from build123d import *

# Parameters (mm, degrees)
SKETCH1_W                                     = 127
SKETCH1_H                                     = 190.5
BOSS_EXTRUDE1_DEPTH                           = 16
SKETCH3_W                                     = 73.2
SKETCH3_H                                     = 190.5
CUT_EXTRUDE2_DEPTH                            = 14
SKETCH6_W                                     = 73.2
SKETCH6_H                                     = 120.5
SKETCH6_H_2                                   = 11.470358649
SKETCH6_H_3                                   = 11.529641351
BOSS_EXTRUDE5_DEPTH                           = 14
SKETCH9_W                                     = 49.3
SKETCH9_H                                     = 49.3
SKETCH9_W_2                                   = 43.3
SKETCH9_H_2                                   = 43.3
BOSS_EXTRUDE7_DEPTH                           = 26.9
SKETCH9_5_W                                   = 43.3
SKETCH9_5_H                                   = 43.3
SKETCH9_5_W_2                                 = 31.3
SKETCH9_5_H_2                                 = 31.3
SKETCH9_5_R                                   = 12
BOSS_EXTRUDE8_DEPTH                           = 3
SKETCH10_W                                    = 43.3
SKETCH10_H                                    = 43.3
BOSS_EXTRUDE11_DEPTH                          = 26.9
SKETCH10_5_W                                  = 43.3
SKETCH10_5_H                                  = 43.3
SKETCH10_5_W_2                                = 31.3
SKETCH10_5_H_2                                = 31.3
SKETCH10_5_R                                  = 12
BOSS_EXTRUDE12_DEPTH                          = 3
SKETCH12_R                                    = 1.5
CUT_EXTRUDE4_DEPTH                            = 124
SKETCH13_W                                    = 26.9
SKETCH13_H                                    = 23.5
SKETCH13_H_2                                  = 23.559282703
SKETCH13_H_3                                  = 23.440717297
BOSS_EXTRUDE13_DEPTH                          = 13
CBORE_FOR_M4_PAN_HEAD_MACHINE_SCREW1_AT_COUNT = 2
CBORE_FOR_M4_PAN_HEAD_MACHINE_SCREW1_AT_PITCH = 13.45
CBORE_FOR_M4_PAN_HEAD_MACHINE_SCREW1_2_COUNT  = 2
CBORE_FOR_M4_PAN_HEAD_MACHINE_SCREW1_2_PITCH  = 86.65000507
CBORE_FOR_M4_PAN_HEAD_MACHINE_SCREW1_3_COUNT  = 2
CBORE_FOR_M4_PAN_HEAD_MACHINE_SCREW1_3_PITCH  = 100.100004389
CBORE_FOR_M4_PAN_HEAD_MACHINE_SCREW1_4_COUNT  = 2
CBORE_FOR_M4_PAN_HEAD_MACHINE_SCREW1_4_PITCH  = 167.16209619
CBORE_FOR_M4_PAN_HEAD_MACHINE_SCREW1_5_COUNT  = 2
CBORE_FOR_M4_PAN_HEAD_MACHINE_SCREW1_5_PITCH  = 159.472188492
CBORE_FOR_M4_PAN_HEAD_MACHINE_SCREW1_6_COUNT  = 2
CBORE_FOR_M4_PAN_HEAD_MACHINE_SCREW1_6_PITCH  = 133.877393172
CBORE_FOR_M4_PAN_HEAD_MACHINE_SCREW1_7_COUNT  = 2
CBORE_FOR_M4_PAN_HEAD_MACHINE_SCREW1_7_PITCH  = 134.551324417
CUT_EXTRUDE8_START                            = -127
SKETCH27_R                                    = 5
CUT_EXTRUDE8_DEPTH                            = 127
SPLIT1_SURFACE_1_BACK                         = 278.18
SPLIT1_SURFACE_1_DEPTH                        = 556.36


with BuildPart() as part:
    # Sketch1 → Boss-Extrude1 (new body)
    with BuildSketch(Plane(origin=(0, 0, 0), x_dir=(1, 0, 0), z_dir=(0, 1, 0))):
        with Locations((22.032491394, 64.602312685)):
            Rectangle(SKETCH1_W, SKETCH1_H)
    extrude(amount=BOSS_EXTRUDE1_DEPTH)

    # Sketch3 → Cut-Extrude2 (cut)
    with BuildSketch(Plane(origin=(0, 16, 0), x_dir=(1, 0, 0), z_dir=(0, 1, 0))):
        with Locations((22.032491394, 64.602312685)):
            Rectangle(SKETCH3_W, SKETCH3_H)
    extrude(amount=-CUT_EXTRUDE2_DEPTH, mode=Mode.SUBTRACT)

    # Sketch6 → Boss-Extrude5 (add)
    with BuildSketch(Plane(origin=(0, 2, 0), x_dir=(1, 0, 0), z_dir=(0, 1, 0))):
        with Locations((22.032491394, 64.631954036)):
            Rectangle(SKETCH6_W, SKETCH6_H)
        with Locations((22.032491394, 154.117133361)):
            Rectangle(SKETCH6_W, SKETCH6_H_2)
        with Locations((22.032491394, -24.88286664)):
            Rectangle(SKETCH6_W, SKETCH6_H_3)
    extrude(amount=BOSS_EXTRUDE5_DEPTH)

    # Sketch9 → Boss-Extrude7 (add)
    with BuildSketch(Plane.ZY.offset(41.467508606)):
        Polygon((-77.781954036, 106.934621953), (-89.252312685, 106.934621953), (-159.852312685, 16), (-148.381954036, 16), align=None)
        with Locations((-64.602312685, 131.584621953)):
            Rectangle(SKETCH9_W, SKETCH9_H)
        with Locations((-64.602312685, 131.584621953)):
            Rectangle(SKETCH9_W_2, SKETCH9_H_2, mode=Mode.SUBTRACT)
        Polygon((30.647687315, 16), (-39.952312685, 106.934621953), (-51.481954036, 106.934621953), (19.118045964, 16), align=None)
    extrude(amount=-BOSS_EXTRUDE7_DEPTH)

    # Sketch9<5> → Boss-Extrude8 (add)
    with BuildSketch(Plane.ZY.offset(41.467508606)):
        with Locations((-64.602312685, 131.584621953)):
            Rectangle(SKETCH9_5_W, SKETCH9_5_H)
        with Locations((-64.602312685, 131.584621953)):
            Rectangle(SKETCH9_5_W_2, SKETCH9_5_H_2, mode=Mode.SUBTRACT)
        with Locations((-64.602312685, 131.584621953)):
            Rectangle(SKETCH9_5_W_2, SKETCH9_5_H_2)
        with Locations((-64.602312685, 131.584621953)):
            Circle(SKETCH9_5_R, mode=Mode.SUBTRACT)
    extrude(amount=-BOSS_EXTRUDE8_DEPTH)

    # Sketch10 → Boss-Extrude11 (add)
    with BuildSketch(Plane(origin=(85.532491394, 0, 0), x_dir=(0, 0, -1), z_dir=(1, 0, 0))):
        Polygon((89.192671333, 156.174980602), (39.952312685, 156.174980602), (39.952312685, 106.934621953), (-30.647687315, 16), (-19.177328667, 16), (51.422671333, 106.934621953), (77.722671333, 106.934621953), (148.322671333, 16), (159.792671333, 16), (89.192671333, 106.934621953), align=None)
        with Locations((64.602312685, 131.584621953)):
            Rectangle(SKETCH10_W, SKETCH10_H, mode=Mode.SUBTRACT)
    extrude(amount=-BOSS_EXTRUDE11_DEPTH)

    # Sketch10<5> → Boss-Extrude12 (add)
    with BuildSketch(Plane(origin=(85.532491394, 0, 0), x_dir=(0, 0, -1), z_dir=(1, 0, 0))):
        with Locations((64.602312685, 131.584621953)):
            Rectangle(SKETCH10_5_W, SKETCH10_5_H)
        with Locations((64.602312685, 131.584621953)):
            Rectangle(SKETCH10_5_W_2, SKETCH10_5_H_2, mode=Mode.SUBTRACT)
        with Locations((64.602312685, 131.584621953)):
            Rectangle(SKETCH10_5_W_2, SKETCH10_5_H_2)
        with Locations(Location((64.602312685, 131.584621953, 0), (0, 0, 180))):
            Circle(SKETCH10_5_R, mode=Mode.SUBTRACT)
    extrude(amount=-BOSS_EXTRUDE12_DEPTH)

    # Sketch12 → Cut-Extrude4 (cut)
    with BuildSketch(Plane(origin=(-38.467508606, 0, 0), x_dir=(0, 0, -1), z_dir=(1, 0, 0))):
        with Locations(Location((80.102312685, 147.084621953, 0), (0, 0, 180))):
            Circle(SKETCH12_R)
        with Locations(Location((49.102312685, 147.084621953, 0), (0, 0, 180))):
            Circle(SKETCH12_R)
        with Locations(Location((49.102312685, 116.084621953, 0), (0, 0, 180))):
            Circle(SKETCH12_R)
        with Locations(Location((80.102312685, 116.084621953, 0), (0, 0, 180))):
            Circle(SKETCH12_R)
    extrude(amount=CUT_EXTRUDE4_DEPTH, mode=Mode.SUBTRACT)

    # Sketch13 → Boss-Extrude13 (add)
    with BuildSketch(Plane(origin=(0, 16, 0), x_dir=(1, 0, 0), z_dir=(0, 1, 0))):
        with Locations((-28.017508606, 136.631954036)):
            Rectangle(SKETCH13_W, SKETCH13_H)
        with Locations((-28.017508606, -7.368045964)):
            Rectangle(SKETCH13_W, SKETCH13_H)
        with Locations((72.082491394, -7.397687316)):
            Rectangle(SKETCH13_W, SKETCH13_H_2)
        with Locations((72.082491394, 136.602312685)):
            Rectangle(SKETCH13_W, SKETCH13_H_3)
    extrude(amount=BOSS_EXTRUDE13_DEPTH)

    # Sketch24 → CBORE for M4 Pan Head Machine Screw1 (revolve, cut)
    with BuildSketch(Plane(origin=(-21.292508606, 0, 2.321563226), x_dir=(0, 0, -1), z_dir=(1, 0, 0))):
        Polygon((0, 0), (0, 26.291850331), (2.15, 25), (2.15, 3.1), (4.5, 3.1), (4.5, 0.046044272), (4.525, 0), align=None)
    cbore_for_m4_pan_head_machine_screw1 = revolve(axis=Axis((-21.292508606, -6.35, 2.321563226), (0, 1, 0)), mode=Mode.SUBTRACT)

    # CBORE for M4 Pan Head Machine Screw1 at: CBORE for M4 Pan Head Machine Screw1 ×2
    with Locations(*[(-i * CBORE_FOR_M4_PAN_HEAD_MACHINE_SCREW1_AT_PITCH, 0, 0) for i in range(1, CBORE_FOR_M4_PAN_HEAD_MACHINE_SCREW1_AT_COUNT)]):
        add(cbore_for_m4_pan_head_machine_screw1, mode=Mode.SUBTRACT)

    # CBORE for M4 Pan Head Machine Screw1 2: CBORE for M4 Pan Head Machine Screw1 ×2
    with Locations(*[Vector(0.9999999414901701, 0, 0.00034208135925630124) * (i * CBORE_FOR_M4_PAN_HEAD_MACHINE_SCREW1_2_PITCH) for i in range(1, CBORE_FOR_M4_PAN_HEAD_MACHINE_SCREW1_2_COUNT)]):
        add(cbore_for_m4_pan_head_machine_screw1, mode=Mode.SUBTRACT)

    # CBORE for M4 Pan Head Machine Screw1 3: CBORE for M4 Pan Head Machine Screw1 ×2
    with Locations(*[Vector(0.9999999561572464, 0, 0.0002961173847583374) * (i * CBORE_FOR_M4_PAN_HEAD_MACHINE_SCREW1_3_PITCH) for i in range(1, CBORE_FOR_M4_PAN_HEAD_MACHINE_SCREW1_3_COUNT)]):
        add(cbore_for_m4_pan_head_machine_screw1, mode=Mode.SUBTRACT)

    # CBORE for M4 Pan Head Machine Screw1 4: CBORE for M4 Pan Head Machine Screw1 ×2
    with Locations(*[Vector(0.5988199614729853, 0, -0.8008836705424156) * (i * CBORE_FOR_M4_PAN_HEAD_MACHINE_SCREW1_4_PITCH) for i in range(1, CBORE_FOR_M4_PAN_HEAD_MACHINE_SCREW1_4_COUNT)]):
        add(cbore_for_m4_pan_head_machine_screw1, mode=Mode.SUBTRACT)

    # CBORE for M4 Pan Head Machine Screw1 5: CBORE for M4 Pan Head Machine Screw1 ×2
    with Locations(*[Vector(0.5433549311591849, 0, -0.8395030784845268) * (i * CBORE_FOR_M4_PAN_HEAD_MACHINE_SCREW1_5_PITCH) for i in range(1, CBORE_FOR_M4_PAN_HEAD_MACHINE_SCREW1_5_COUNT)]):
        add(cbore_for_m4_pan_head_machine_screw1, mode=Mode.SUBTRACT)

    # CBORE for M4 Pan Head Machine Screw1 6: CBORE for M4 Pan Head Machine Screw1 ×2
    with Locations(*[(0, 0, -i * CBORE_FOR_M4_PAN_HEAD_MACHINE_SCREW1_6_PITCH) for i in range(1, CBORE_FOR_M4_PAN_HEAD_MACHINE_SCREW1_6_COUNT)]):
        add(cbore_for_m4_pan_head_machine_screw1, mode=Mode.SUBTRACT)

    # CBORE for M4 Pan Head Machine Screw1 7: CBORE for M4 Pan Head Machine Screw1 ×2
    with Locations(*[Vector(-0.09996185513764777, 0, -0.9949912700709691) * (i * CBORE_FOR_M4_PAN_HEAD_MACHINE_SCREW1_7_PITCH) for i in range(1, CBORE_FOR_M4_PAN_HEAD_MACHINE_SCREW1_7_COUNT)]):
        add(cbore_for_m4_pan_head_machine_screw1, mode=Mode.SUBTRACT)

    # Sketch27 → Cut-Extrude8 (cut)
    with BuildSketch(Plane.ZY.offset(41.467508606).offset(CUT_EXTRUDE8_START)):
        with Locations((-142.36713336, 8)):
            Circle(SKETCH27_R)
        with Locations((13.13286664, 8.093964388)):
            Circle(SKETCH27_R)
    extrude(amount=CUT_EXTRUDE8_DEPTH, mode=Mode.SUBTRACT)

    # Split1: cut with a surface, the side it looks to stays
    # Split1 surface: a surface, the sketch's curves swept straight by 556.36 mm
    with BuildLine(Plane.XY.offset(30.647687315).offset(-SPLIT1_SURFACE_1_BACK), mode=Mode.PRIVATE) as split1_surface_1_path:
        Line((-14.567508606, 16), (-14.567508606, 0))
    split1_surface_1 = Shell.extrude(split1_surface_1_path.wire(), (0 * SPLIT1_SURFACE_1_DEPTH, 0 * SPLIT1_SURFACE_1_DEPTH, 1 * SPLIT1_SURFACE_1_DEPTH))
    split(bisect_by=split1_surface_1, keep=Keep.TOP)


solid = part.part
Design review of the part built by this model. Coordinates are the model's own, in mm. A direction names the side the tool comes from. Give positions to 0.01 mm unless a question says otherwise; leave off trailing zeros. Write each loop counter-clockwise with the first axis right and the second up, starting at its lowest first coordinate (ties: lowest second). Pieces come first, ordered by that corner, then holes. Notation, with made-up numbers: M 39.25,34 L 95.25,34 A12 cw 95.25,39 Z; hole C 53.5,-28.75 d4. An arc over 180 degrees is marked long. Return JSON: item names as keys, results as strings. Group by question number.
Item 1: Tool access review of faces 5 (the flat face through (81, 3.1, -133)), 6 (the flat face through (-14.568, 8, -87)), 7 (the flat face through (22, 9, 19.118)), 8 (the flat face through (72, 22, -4.382)), 9 (the flat face through (71, 131, -86.252)): name each direction out of +Z, -Z, +X, -X, +Y, -Y from which nothing blocks a thin tool from reaching the whole face with its end or side.
Item 2: Take a section at A-A (x = 27.5). Give the boundary of the cut face in (y, z), plus the area to 3 significant figures.
Item 3: Take a section at B-B (z = -142.5). Give the boundary of the cut face in (x, y).
Item 4: Wall thickness on line 1 along Z through (x, y) = (35.5, 12.5); line 2 along Y through (x, z) = (68, -44.5); line 3 along Z through (x, y) = (63, 138): over which ranges is each line inside the solid? List them lowest first.
Item 5: Clearance check with flat-ended pins moving along their axes: pin 1 Ø12 at (x, z) = (19.5, 10) entering from +Y; pin 2 Ø4 at (x, z) = (18, -84) entering from +Y; pin 3 Ø21.5 at (x, y) = (72.5, 119.5) entering from +Z. State where each tip first meets the part, or that it passes through.
Item 6: The part is to be moulded in two halves that separate along Y. For faces 1 (the flat face through (85.532, 90, -92)), 2 (the flat face through (63, 3.1, 3)), 3 (the cylindrical face through (72.271, 9.502, -137.598)), 4 (the flat face through (72, 29, 2)), say which applies: pulls with the +Y half, pulls with the -Y half, needs draft (parallel to the pull), parting line crosses it, or undercut.
Return value:
{
 "1": {"face 5": "-Y", "face 6": "+Z, -Z, -X, +Y, -Y", "face 7": "-X, +Y", "face 8": "+X, -X", "face 9": "-X"},
 "2": {"outline": "M 0,-159.85 L 16,-159.85 L 16,-148.38 L 2,-148.38 L 2,-124.88 L 16,-124.88 L 16,-4.38 L 2,-4.38 L 2,19.12 L 16,19.12 L 16,30.65 L 0,30.65 Z", "area": "2,390 mm2"},
 "3": {"outline": "M -14.57,0 L 85.53,0 L 85.53,3 L 58.63,3 L 58.63,2 L -14.57,2 Z; M 58.63,13 L 85.53,13 L 85.53,38.27 L 58.63,38.27 Z"},
 "4": {"line 1": "z = -159.85 to -148.38, -124.88 to -4.38, 19.12 to 30.65", "line 2": "y = 0 to 16, 98.02 to 109.93, 153.23 to 156.17", "line 3": "z = -89.19 to -86.25, -42.95 to -39.95"},
 "5": {"pin 1": "stops at y = 2", "pin 2": "stops at y = 16", "pin 3": "stops at z = -39.95"},
 "6": {"face 1": "needs draft", "face 2": "pulls with the -Y half", "face 3": "undercut", "face 4": "undercut"}
}
